Geometry check sheet. Reference: drawing and pictorial views, mm from the part's lowest x, y, z. A direction names the side the tool comes from. Round coordinates to 2 decimals unless told otherwise and drop trailing zeros. Write each loop counter-clockwise with the first axis right and the second up, starting at its lowest first coordinate (ties: lowest second). Pieces come first, ordered by that corner, then holes. Notation, with made-up numbers: (89, 39) - (135, 39) arc R18 cw to (135, 62) - close; hole circle Ø4 at (7.25, 15.5). An arc over 180 degrees is marked (long way). Return JSON: item names as keys, results as strings.
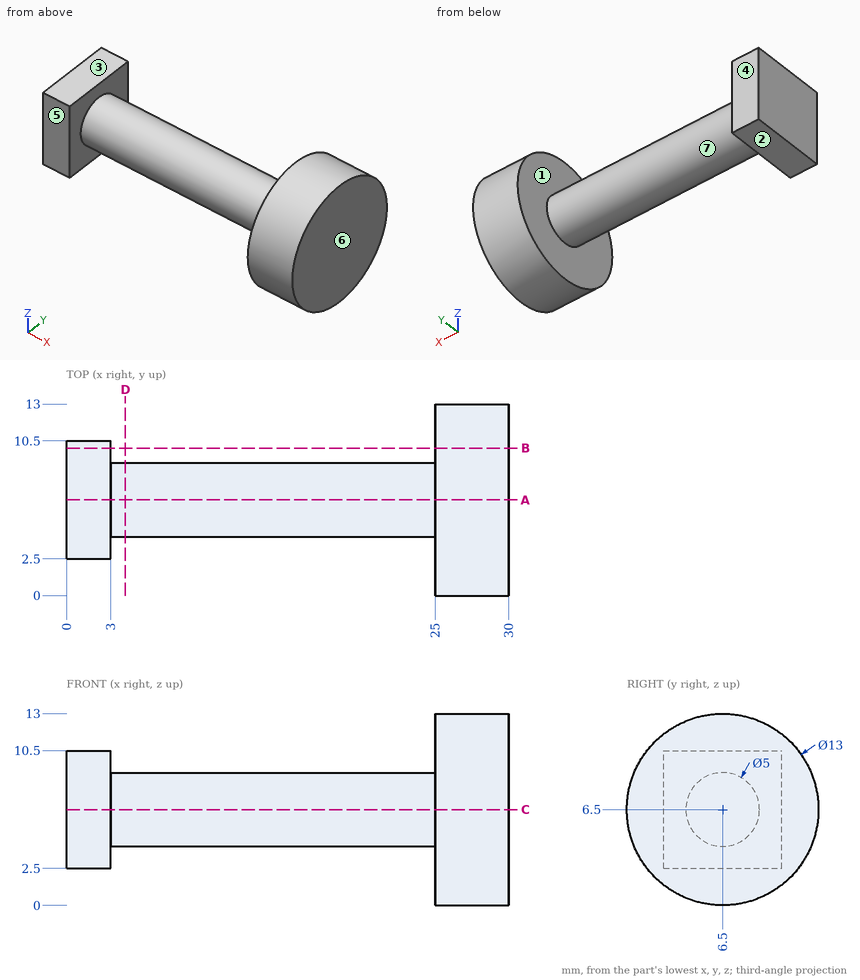
(1) Access from +Z, -Z, +X, -X, +Y, -Y to the whole of each face (thin tool, end or side, straight path). Record for the marked faces 1, 2, 3 and 4.
Response values:
{"face 1": "none", "face 2": "-Z, -X, +Y, -Y", "face 3": "+Z, -X, +Y, -Y", "face 4": "+Z, -Z, -X, +Y"}
(2) Gauge pin test, flat ends, axial feed: pin 1 (0.9 mm diameter, centred on x = 1, y = 4.5, fed in from -Z); pin 2 (5 mm diameter, centred on x = 10.5, z = 3.5, fed in from -Y); pin 3 (3.5 mm diameter, centred on x = 1, z = 6, fed in from +Y). Record the tip position at first contact, or that the pin passes through.
Response values:
{"pin 1": "stops at z = 2.5", "pin 2": "stops at y = 4.05", "pin 3": "stops at y = 10.5"}
(3) Release check for a two-part mould opening along X. For the marked faces 5, 6 and 7 record: pulls with the +X half, pulls with the -X half, needs draft (parallel to the pull), parting line crosses it, or undercut.
Response values:
{"face 5": "needs draft", "face 6": "pulls with the +X half", "face 7": "undercut"}
(4) Section check A-A, the plane y = 6.5. Enter the section's corners in (x, z).
Response values:
{"outline": "(0, 2.5) - (3, 2.5) - (3, 4) - (25, 4) - (25, 0) - (30, 0) - (30, 13) - (25, 13) - (25, 9) - (3, 9) - (3, 10.5) - (0, 10.5) - close"}
(5) Section check B-B, the plane y = 10. Enter the section's corners in (x, z).
Response values:
{"outline": "(0, 2.5) - (3, 2.5) - (3, 10.5) - (0, 10.5) - close; (25, 1.02) - (30, 1.02) - (30, 11.98) - (25, 11.98) - close"}
(6) Material ranges on line 1 along X through (y, z) = (10.25, 9.5); line 2 along X through (y, z) = (6.25, 1.75); line 3 along Z through (x, y) = (1.75, 2.75), recorded low to high. Write a range as [from, to].
Response values:
{"line 1": "x = [0, 3], [25, 30]", "line 2": "x = [25, 30]", "line 3": "z = [2.5, 10.5]"}
(7) Section check D-D, the plane x = 4. Enter the section's corners in (y, z), plus the area to 3 significant figures.
Response values:
{"outline": "circle Ø5 at (6.5, 6.5)", "area": "19.6 mm^2"}
